```python
from build123d import *

# Parameters (mm, degrees)
F0_R     = 50.8
F1_DEPTH = 12.7
F2_R     = 38.1
F3_DEPTH = 57.15
F4_R     = 63.5
F5_DEPTH = 12.7
F6_W     = 50.8
F6_H     = 50.8
F7_DEPTH = 112.776
F8_R     = 6.35
F9_DEPTH = 25.4
F10_R    = 5.08


with BuildPart() as f1:
    # F0 (on Top) → F1 (new body)
    with BuildSketch(Plane.XY):
        Circle(F0_R)
    extrude(amount=F1_DEPTH)

    # F2 (on face) → F3 (join)
    with BuildSketch(Plane.XY):
        Circle(F2_R)
    extrude(amount=-F3_DEPTH)

    # F4 (on face) → F5 (join)
    with BuildSketch(Plane(origin=(0, 0, -57.15), x_dir=(1, 0, 0), z_dir=(0, 0, -1))):
        Circle(F4_R)
    extrude(amount=F5_DEPTH)

    # F6 (on face) → F7 (cut)
    with BuildSketch(Plane.XY.offset(12.7)):
        Rectangle(F6_W, F6_H)
    extrude(amount=-F7_DEPTH, mode=Mode.SUBTRACT)

    # F8 (on face) → F9 (cut)
    with BuildSketch(Plane.XY.offset(-57.15)):
        with Locations((0, -50.8)):
            Circle(F8_R)
        with Locations((50.8, 0)):
            Circle(F8_R)
        with Locations((0, 50.8)):
            Circle(F8_R)
        with Locations((-50.8, 0)):
            Circle(F8_R)
    extrude(amount=-F9_DEPTH, mode=Mode.SUBTRACT)

    # F10
    f10_edges = [f1.edges().sort_by_distance(p)[0] for p in [
        (50.8, 0, 6.35),
        (-50.8, 0, 0),
        (-50.8, 0, 12.7),
    ]]
    fillet(f10_edges, radius=F10_R)


solid = f1.part
```
Could you check a few things on this model? Use its own coordinates, in mm. A direction names the side the tool comes from. Round coordinates to 2 decimals unless told otherwise and drop trailing zeros. Write each loop counter-clockwise with the first axis right and the second up, starting at its lowest first coordinate (ties: lowest second). Pieces come first, ordered by that corner, then holes. Notation, with made-up numbers: M 4.25,-2 L 25.25,-2 A18 cw 25.25,10 Z; hole C 10.5,87.25 d9. An arc over 180 degrees is marked long. Write each question's results on one line, items separated by ' | '. Start each with the question number.
1. I need wall thicknesses on L1, parallel to Y at x = 0, z = -63.5; L2, parallel to Y at x = -50.8, z = -67; L3, parallel to X at y = 8, z = -62.5. Which ranges of each line are inside material? Lowest first, please. Write a range as from..to.
2. Imagine slicing it at D-D on y = -47.5. Count the separate pieces of the cut face and the enclosed holes in it, and give its area (3 significant figures).
3. Imagine slicing it at A-A on x = 0. List the corners of the cut face in (y, z) for me, and give its area (3 significant figures).
4. Thinking about a two-plate mould opening in Y: for faces 4 (the face through (25.4, 0, -28)), 5 (the face through (-11.012, -49.592, 6.332)), 6 (the face through (27.3, 27.3, -57.15)), which applies, +Y half, -Y half, draft (parallel to the pull), parting line (faces both ways), or undercut?
5. Imagine slicing it at C-C on z = -50. List the corners of the cut face in (x, y) for me.
6. On a 3-axis mill with a long thin cutter (end or side, diameter ignored), from which of +Z, -Z, +X, -X, +Y, -Y can I reach the whole of each face in a straight line? I mean faces 1 (the face through (-44.743, 1.907, -63.411)), 2 (the face through (-25.4, 0, -28)), 3 (the face through (-10, 37, 0)). Say none if no direction works.
7. I'm going to push flat-ended pins straight in: pin 1 Ø15 at (x, z) = (-8, -34.5) entering from -Y; pin 2 Ø5 at (x, z) = (21, -30.5) entering from +Y; pin 3 Ø1.5 at (y, z) = (-22.5, -46) entering from +X; pin 4 Ø11.5 at (x, y) = (0, -50.8) entering from +Z. Where does each tip first touch, or does it pass through?
Result sheet:
1) L1: y = -63.5..-57.15, -44.45..-25.4, 25.4..44.45, 57.15..63.5 | L2: y = -38.1..-6.35, 6.35..38.1 | L3: x = -62.99..-25.4, 25.4..62.99
2) separate pieces: 3 | enclosed holes: 0 | area: 1,310 mm^2
3) outline: M -63.5,-69.85 L -57.15,-69.85 L -57.15,-57.15 L -63.5,-57.15 Z; M -50.8,5.08 A5.08 ccw -45.72,0 L -38.1,0 L -38.1,-57.15 L -44.45,-57.15 L -44.45,-69.85 L -25.4,-69.85 L -25.4,12.7 L -45.72,12.7 A5.08 ccw -50.8,7.62 Z; M 25.4,-69.85 L 44.45,-69.85 L 44.45,-57.15 L 38.1,-57.15 L 38.1,0 L 45.72,0 A5.08 ccw 50.8,5.08 L 50.8,7.62 A5.08 ccw 45.72,12.7 L 25.4,12.7 Z; M 57.15,-69.85 L 63.5,-69.85 L 63.5,-57.15 L 57.15,-57.15 Z | area: 2,720 mm^2
4) face 4: undercut | face 5: parting line | face 6: draft
5) outline: C 0,0 d76.2; hole M -25.4,-25.4 L 25.4,-25.4 L 25.4,25.4 L -25.4,25.4 Z
6) face 1: -Z | face 2: +Z, -Z | face 3: none
7) pin 1: stops at y = -38.1 | pin 2: stops at y = 33.31 | pin 3: stops at x = 31.28 | pin 4: stops at z = 12.7
